```python
from build123d import *

# Parameters (mm, degrees)
SKETCH1_R                            = 121.5
SKETCH1_R_2                          = 93.5
SKETCH1_R_3                          = 4.2164
BOSS_EXTRUDE1_DEPTH                  = 6.35
STOPING_SCREW_5_16_18_TAPPED_HOLE1_D = 6.5278
STOP_SCREW_CIRPATTERN1_COUNT         = 8
F_5_16_18_TAPPED_HOLE1_OUTLINE_R     = 3.2639
F_5_16_18_TAPPED_HOLE1_DEPTH         = 6.35
CIRPATTERN1_COUNT                    = 8


# Read off the part's stored shape, not the designer's step: 5/16-18 Tapped Hole1
with BuildPart() as part:
    # Sketch1 → Boss-Extrude1 (new body)
    with BuildSketch(Plane(origin=(0, 0, 0), x_dir=(1, 0, 0), z_dir=(0, 1, 0))):
        with Locations(Location((0, 0, 0), (0, 0, 270))):
            Circle(SKETCH1_R)
        with Locations(Location((0, 0, 0), (0, 0, 270))):
            Circle(SKETCH1_R_2, mode=Mode.SUBTRACT)
        with Locations(Location((0, 100, 0), (0, 0, 270))):
            Circle(SKETCH1_R_3, mode=Mode.SUBTRACT)
        with Locations(Location((70.710678119, 70.710678119, 0), (0, 0, 270))):
            Circle(SKETCH1_R_3, mode=Mode.SUBTRACT)
        with Locations(Location((100, 0, 0), (0, 0, 270))):
            Circle(SKETCH1_R_3, mode=Mode.SUBTRACT)
        with Locations(Location((70.710678119, -70.710678119, 0), (0, 0, 270))):
            Circle(SKETCH1_R_3, mode=Mode.SUBTRACT)
        with Locations(Location((0, -100, 0), (0, 0, 270))):
            Circle(SKETCH1_R_3, mode=Mode.SUBTRACT)
        with Locations(Location((-70.710678119, -70.710678119, 0), (0, 0, 270))):
            Circle(SKETCH1_R_3, mode=Mode.SUBTRACT)
        with Locations(Location((-100, 0, 0), (0, 0, 270))):
            Circle(SKETCH1_R_3, mode=Mode.SUBTRACT)
        with Locations(Location((-70.710678119, 70.710678119, 0), (0, 0, 270))):
            Circle(SKETCH1_R_3, mode=Mode.SUBTRACT)
    extrude(amount=BOSS_EXTRUDE1_DEPTH)

    # Stoping_Screw_5/16-18 Tapped Hole1 (through all)
    with Locations(Plane(origin=(41.329810695, 6.35, 99.778989511), x_dir=(0, 0, 1), z_dir=(0, 1, 0))):
        with Locations((0, 0)):
            stoping_screw_5_16_18_tapped_hole1 = Hole(STOPING_SCREW_5_16_18_TAPPED_HOLE1_D / 2)

    # Stop_Screw_CirPattern1: Stoping_Screw_5/16-18 Tapped Hole1 ×8 about axis
    stop_screw_cirpattern1_axis = Axis((0, 0, 0), (0, 1, 0))
    for i in range(1, STOP_SCREW_CIRPATTERN1_COUNT):
        add(stoping_screw_5_16_18_tapped_hole1.rotate(stop_screw_cirpattern1_axis, i * 360 / STOP_SCREW_CIRPATTERN1_COUNT), mode=Mode.SUBTRACT)

    # 5/16-18 Tapped Hole1 outline → 5/16-18 Tapped Hole1 (cut)
    with BuildSketch(Plane(origin=(0, 0, 0), x_dir=(1, 0, 0), z_dir=(0, 1, 0))):
        with Locations((58.028357701, -91.086276148)):
            Circle(F_5_16_18_TAPPED_HOLE1_OUTLINE_R)
        with Locations((23.375478305, -105.439968769)):
            Circle(F_5_16_18_TAPPED_HOLE1_OUTLINE_R)
    f_5_16_18_tapped_hole1 = extrude(amount=F_5_16_18_TAPPED_HOLE1_DEPTH, mode=Mode.SUBTRACT)

    # CirPattern1: 5/16-18 Tapped Hole1 ×8 about axis
    cirpattern1_axis = Axis((0, 0, 0), (0, 1, 0))
    for i in range(1, CIRPATTERN1_COUNT):
        add(f_5_16_18_tapped_hole1.rotate(cirpattern1_axis, i * 360 / CIRPATTERN1_COUNT), mode=Mode.SUBTRACT)


solid = part.part
```
Read the model definition and answer for the solid it produces. Units are mm, in the model's axes. Give positions to 0.01 mm unless a question says otherwise; leave off trailing zeros. Order: outer loops, then holes, each group sorted by start corner. A loop starts at its lowest first (then second) coordinate and runs counter-clockwise, first axis right, second up.
(1) Find section D-D (y = 4.75). Give the number of separate pieces and of enclosed holes in the cut face, plus the area to 3 significant figures.
(2) Straight lines are drawn through the part: L1, parallel to X at y = 0.75, z = 61; L2, parallel to Z at x = 74, y = 5.25; L3, parallel to X at y = 6.25, z = -41. For each, find the intervals that lie inside material, in ascending order.
(3) Given pin 1 (8.5 mm diameter, centred on x = -91.09, z = 58.03, fed in from +Y), flat-ended and moving along its own axis, determine where the tip first touches the part or whether it passes through.
(4) Find section C-C (x = 83). Give the vertices of the cut face in (y, z).
(5) Find section B-B (x = 0). Give the vertices of the cut face in (y, z), plus the area to 3 significant figures.
(6) For a pull along Z with two mould halves and no side action, classify faces 1 (the cylindrical face through (-118.61, 3.13, -26.34)), 2 (the cylindrical face through (-41.47, 3.13, -103.04)), 3 (the flat face through (-71, 6.35, 62)) as released by +Z, released by -Z, zero draft, split by the parting line, or undercut.
(7) Find section A-A (z = -13.5). Give the vertices of the cut face in (x, y).
Result sheet:
1. separate pieces: 1
1. enclosed holes: 33
1. area: 17,700 mm2
2. L1: x = -105.08 to -92.44, -89.74 to -70.86, 70.86 to 89.74, 92.44 to 105.08
2. L2: z = -96.37 to -73.35, -68.07 to -57.15, 57.15 to 68.07, 73.35 to 96.37
2. L3: x = -114.37 to -103.03, -96.53 to -84.03, 84.03 to 96.53, 103.03 to 114.37
3. pin 1: stops at y = 6.35
4. outline: (0, -88.73) - (6.35, -88.73) - (6.35, -43.05) - (0, -43.05) - close; (0, 43.05) - (6.35, 43.05) - (6.35, 88.73) - (0, 88.73) - close
5. outline: (0, -121.5) - (6.35, -121.5) - (6.35, -104.22) - (0, -104.22) - close; (0, -95.78) - (6.35, -95.78) - (6.35, -93.5) - (0, -93.5) - close; (0, 93.5) - (6.35, 93.5) - (6.35, 95.78) - (0, 95.78) - close; (0, 104.22) - (6.35, 104.22) - (6.35, 121.5) - (0, 121.5) - close
5. area: 249 mm2
6. face 1: split by the parting line
6. face 2: undercut
6. face 3: zero draft
7. outline: (-120.75, 0) - (-92.52, 0) - (-92.52, 6.35) - (-120.75, 6.35) - close; (92.52, 0) - (120.75, 0) - (120.75, 6.35) - (92.52, 6.35) - close
